Source: CAD feature listing. Evaluate the final solid. Frame: model axes, mm. A direction names the side the tool comes from. Give positions to 0.01 mm unless a question says otherwise; leave off trailing zeros. Order: outer loops, then holes, each group sorted by start corner. A loop starts at its lowest first (then second) coordinate and runs counter-clockwise, first axis right, second up.
from build123d import *

# Parameters (mm, degrees)
F7_DEPTH      = 1.5875
F7_DEPTH_BACK = 1.5875
F8_R          = 3.175
F9_DEPTH      = 3.175


with BuildPart() as f2:
    # F2: sweep along a path in F0
    with BuildLine(Plane.XZ) as f2_path:
        Line((876.3, 0), (756.8278850907, 375.134780791))
        Line((756.8278850907, 375.134780791), (609.9778582309, 533.4))
        Line((609.9778582309, 533.4), (0, 533.4))
        Line((0, 533.4), (-609.9778582309, 533.4))
        Line((-609.9778582309, 533.4), (-756.8278850907, 375.134780791))
        Line((-756.8278850907, 375.134780791), (-876.3, 0))
        Line((-876.3, 0), (0, 0))
        Line((0, 0), (876.3, 0))
    # F1 (on Top) → F2 (sweep)
    with BuildSketch(Plane.XY):
        Polygon((886.8210244843, 25.4), (865.7789755157, 25.4), (850.9, 10.5210244843), (850.9, -10.5210244843), (865.7789755157, -25.4), (886.8210244843, -25.4), (901.7, -10.5210244843), (901.7, 10.5210244843), align=None)
    sweep(path=f2_path.line, transition=Transition.RIGHT)



with BuildPart() as f4:
    # F4: sweep along a path in F0
    with BuildLine(Plane.XZ) as f4_path:
        Line((187.325, 533.4), (187.325, 0))
    # F3 (on Top) → F4 (sweep)
    with BuildSketch(Plane.XY):
        Polygon((197.8460244843, 25.4), (176.8039755157, 25.4), (161.925, 10.5210244843), (161.925, -10.5210244843), (176.8039755157, -25.4), (197.8460244843, -25.4), (212.725, -10.5210244843), (212.725, 10.5210244843), align=None)
    sweep(path=f4_path.line)


with BuildPart() as f5:
    # F5: sweep along a path in F0
    with BuildLine(Plane.XZ) as f5_path:
        Line((-187.325, 533.4), (-187.325, 0))
    # F3 (on Top) → F5 (sweep)
    with BuildSketch(Plane.XY):
        Polygon((-176.8039755157, 25.4), (-197.8460244843, 25.4), (-212.725, 10.5210244843), (-212.725, -10.5210244843), (-197.8460244843, -25.4), (-176.8039755157, -25.4), (-161.925, -10.5210244843), (-161.925, 10.5210244843), align=None)
    sweep(path=f5_path.line)


with BuildPart() as f2_1:
    add(f2.part)

    add(f4.part)  # F7 merges F4

    add(f5.part)  # F7 merges F5
    # F6 (on Front) → F7 (join, two sides)
    with BuildSketch(Plane.XZ) as f7_sk:
        Polygon((-735.4080395805, 362.6373508831), (-843.1921216188, 24.202243922), (-212.725, 24.202243922), (-212.725, 509.197756078), (-599.4185938449, 509.197756078), align=None)
        Polygon((-808.445752084, 49.602243922), (-712.9281373981, 349.5214298683), (-588.3367571247, 483.797756078), (-238.125, 483.797756078), (-238.125, 49.602243922), align=None, mode=Mode.SUBTRACT)
        Polygon((212.725, 24.202243922), (843.1921216188, 24.202243922), (735.4080395805, 362.6373508831), (599.4185938449, 509.197756078), (212.725, 509.197756078), align=None)
        Polygon((712.9281373981, 349.5214298683), (808.445752084, 49.602243922), (238.125, 49.602243922), (238.125, 483.797756078), (588.3367571247, 483.797756078), align=None, mode=Mode.SUBTRACT)
    extrude(amount=F7_DEPTH)
    extrude(f7_sk.sketch, amount=-F7_DEPTH_BACK)

    # F8 (on face) → F9 (cut, through all)
    with BuildSketch(Plane.XZ.offset(1.5875)):
        with Locations((-225.425, 36.902243922)):
            Circle(F8_R)
        with Locations((-225.425, 496.489843922)):
            Circle(F8_R)
        with Locations((-588.645, 496.489843922)):
            Circle(F8_R)
        with Locations((-725.6281373981, 349.5214298683)):
            Circle(F8_R)
        with Locations((-821.1566, 36.902243922)):
            Circle(F8_R)
        with Locations((225.425, 36.902243922)):
            Circle(F8_R)
        with Locations((225.425, 496.489843922)):
            Circle(F8_R)
        with Locations((588.645, 496.489843922)):
            Circle(F8_R)
        with Locations((725.6281373981, 349.5214298683)):
            Circle(F8_R)
        with Locations((821.1566, 36.902243922)):
            Circle(F8_R)
    extrude(amount=-F9_DEPTH, mode=Mode.SUBTRACT)


solid = f2_1.part
1) Section query B-B on z = 188.5. State how many separate pieces and enclosed holes the cut face has, and give its area (3 significant figures).
Checks:
separate pieces: 4
enclosed holes: 0
area: 8,880 mm2
2) Section query A-A on x = 389. Output: boundary loops of the cut face in (y, z).
Checks:
outline: (-25.4, -10.02) - (-10.52, -24.2) - (10.52, -24.2) - (25.4, -10.02) - (25.4, 10.02) - (10.52, 24.2) - (1.59, 24.2) - (1.59, 49.6) - (-1.59, 49.6) - (-1.59, 24.2) - (-10.52, 24.2) - (-25.4, 10.02) - close; (-25.4, 523.38) - (-10.52, 509.2) - (-1.59, 509.2) - (-1.59, 483.8) - (1.59, 483.8) - (1.59, 509.2) - (10.52, 509.2) - (25.4, 523.38) - (25.4, 543.42) - (10.52, 557.6) - (-10.52, 557.6) - (-25.4, 543.42) - close
3) Pull-direction query (Z, two-part tool) for faces 6 (the face through (788.546, -5.992, 195.789)), 7 (the face through (-830.347, 21.198, 190.519)), 8 (the face through (-194, 25.4, 247)); classes: +Z half, -Z half, draft (parallel to the pull), parting line (faces both ways), or undercut.
Checks:
face 6: undercut
face 7: +Z half
face 8: draft
4) Ray query, L1, parallel to X at y = 15, z = 31; L2, parallel to X at y = -16, z = 476.5; L3, parallel to Z at x = -419.5, y = -10. Return the intervals inside material, ascending.
Checks:
L1: x = -887.35 to -845.51, -208.25 to -166.4, 166.4 to 208.25, 845.51 to 887.35
L2: x = -688.67 to -636.88, -207.25 to -167.4, 167.4 to 207.25, 636.88 to 688.67
L3: z = -24.2 to 24.2, 509.2 to 557.6
5) First-contact query: pin 1 Ø8.5 at (x, z) = (-725.63, 349.52) entering from -Y; pin 2 Ø3 at (y, z) = (12, 49.5) entering from -X; pin 3 Ø10 at (x, z) = (225.42, 496.49) entering from +Y; pin 4 Ø5 at (x, z) = (-588.64, 496.49) entering from +Y. Flat tips, straight axial feed; report the tip coordinate or a pass-through.
Checks:
pin 1: stops at y = -1.59
pin 2: stops at x = -886.03
pin 3: stops at y = 1.59
pin 4: passes through
6) Reachability of faces 1 (the face through (-690.892, 16.674, 473.16)), 2 (the face through (-506, -1.588, 34)), 3 (the face through (693.568, 17.055, 469.741)), 4 (the face through (649.76, -0.02, 417.6)), 5 (the face through (480, 1.588, 34)) from +Z, -Z, +X, -X, +Y, -Y: full face, straight path, thin tool, end or side. Return the list, or none.
Checks:
face 1: +Z, -X, +Y
face 2: -Y
face 3: +Z, +X, +Y
face 4: +Y, -Y
face 5: +Y
